from build123d import *

# Parameters (mm, degrees)
F0_W     = 54.1937425733
F0_H     = 54.301276803
F1_DEPTH = 1003.3
F1_TAPER = 0.7
F2_R     = 4.4355326491
F3_DEPTH = 630.428
F3_TAPER = 1


# Not quite as in the source:
# - a feature names something its author has since deleted; it is built from what else it names


with BuildPart() as f1:
    # F0 (on Top) → F1 (new body)
    with BuildSketch(Plane.XY):
        Rectangle(F0_W, F0_H)
    extrude(amount=F1_DEPTH, taper=F1_TAPER)

    # F2 (on face) → F3 (join)
    with BuildSketch(Plane.XY.offset(1003.3)):
        Circle(F2_R)
    extrude(amount=F3_DEPTH, taper=F3_TAPER)


solid = f1.part
Part model, mm, in its own coordinate system. A direction names the side the tool comes from. Coordinates: 2 decimals unless noted, no trailing zeros. Loops run counter-clockwise (first coordinate to the right, second up) from the corner with the lowest first, then second, coordinate; pieces in that order, holes last. Notation, with made-up numbers: (-16.75, -36) -> (-12.75, -36) arc R6 ccw to (-12.75, -30) -> close; hole circle Ø7 at (57, 31). An arc over 180 degrees is marked (long way). Use a Markdown table: item, result. Add a question column.
Item 1: Band-saw the part on C-C on z = 369. Write the cut outline in (x, y).
Item 2: Probe probe 1 along Z at (x, y) = (11, -5.5); probe 2 along X at (y, z) = (6, 233.5); probe 3 along X at (y, z) = (23.5, 119). List the from-to ranges inside material, lowest first.
Item 3: Flat gauge pins, fed straight in: P1, Ø10, axis at y = 10.5, z = 192, coming from the -X side; P2, Ø3, axis at y = -4, z = 284.5, coming from the +X side; P3, Ø1, axis at y = 4, z = 320.5, coming from the -X side. Where does each tip first touch, or does it go through?
Item 4: Band-saw the part on B-B on z = 1070.5. Write the cut outline in (x, y).
Item 5: Which spindle directions (+Z, -Z, +X, -X, +Y, -Y) get a long thin tool onto all of the face, cutting with end or side? Do faces 1 (the flat face through (0, 0, 0)), 2 (the flat face through (-4, 4, 1003.3)). Say none if no direction does.
Item 6: Band-saw the part on A-A on z = 213. Write the cut outline in (x, y).
Geometry says:
| question | item | result |
|---|---|---|
| 1 | outline | (-22.59, -22.64) -> (22.59, -22.64) -> (22.59, 22.64) -> (-22.59, 22.64) -> close |
| 2 | probe 1 | 0 to 1003.3 |
| 2 | probe 2 | -24.24 to 24.24 |
| 2 | probe 3 | -25.64 to 25.64 |
| 3 | P1 | x = -24.81 |
| 3 | P2 | x = 23.64 |
| 3 | P3 | x = -23.19 |
| 4 | outline | circle Ø6.53 at (0, 0) |
| 5 | face 1 | -Z, +X, -X, +Y, -Y |
| 5 | face 2 | +Z |
| 6 | outline | (-24.49, -24.55) -> (24.49, -24.55) -> (24.49, 24.55) -> (-24.49, 24.55) -> close |
